Source: CAD feature listing. Evaluate the final solid. Frame: model axes, mm. Face numbers are marked on the shaded views. Give positions to 0.01 mm unless a question says otherwise; leave off trailing zeros. Write each loop counter-clockwise with the first axis right and the second up, starting at its lowest first coordinate (ties: lowest second). Pieces come first, ordered by that corner, then holes. Notation, with made-up numbers: (-29.5, 76.25) -> (-6.5, 76.25) arc R31 ccw to (-6.5, 110.25) -> close; hole circle Ø6 at (45.25, 3). An arc over 180 degrees is marked (long way). Write item = value, one per line.
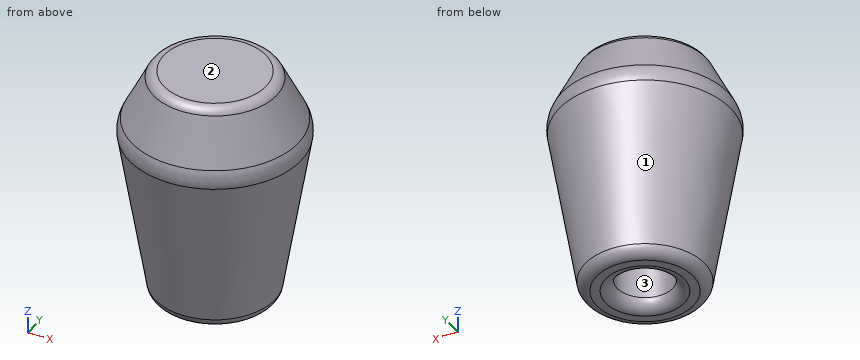
from build123d import *

# Parameters (mm, degrees)
F2_R     = 3.025775
F3_DEPTH = 11.43
F4_R     = 1.27
F5_R     = 3.175


with BuildPart() as f1:
    # F0 (on Front) → F1 (revolve)
    with BuildSketch(Plane.XZ):
        Polygon((0, 25.4), (0, 0), (6.35, 0), (9.525, 19.05), (6.35, 25.4), align=None)
    revolve(axis=Axis((0, 0, 12.7), (0, 0, 1)))

    # F2 (on face) → F3 (cut)
    with BuildSketch(Plane(origin=(0, 0, 0), x_dir=(1, 0, 0), z_dir=(0, 0, -1))):
        Circle(F2_R)
    extrude(amount=-F3_DEPTH, mode=Mode.SUBTRACT)

    # F4
    f4_edges = [f1.edges().sort_by_distance(p)[0] for p in [
        (-3.025775, 0, 0),
        (-6.35, 0, 25.4),
        (-6.35, 0, 0),
    ]]
    fillet(f4_edges, radius=F4_R)

    # F5
    f5_edges = [f1.edges().sort_by_distance(p)[0] for p in [
        (-9.525, 0, 19.05),
    ]]
    fillet(f5_edges, radius=F5_R)


solid = f1.part
(1) Section query B-B (z = 23.5). Return loops of the section in (x, y).
Values follow:
outline = circle Ø14.6 at (0, 0)
(2) Pull-direction query (X, two-part tool) for the marked faces 1, 2 and 3; classes: pulls with the +X half, pulls with the -X half, needs draft (parallel to the pull), parting line crosses it, or undercut.
Values follow:
face_1 = parting line crosses it
face_2 = needs draft
face_3 = undercut
(3) Material intervals for line 1 (X direction, y = 0, z = 5.5); line 2 (Z direction, x = -2.5, y = 1.5); line 3 (X direction, y = 0, z = 3.5), sorted ascending.
Values follow:
line_1 = -7.27 to -3.03, 3.03 to 7.27
line_2 = 11.43 to 25.4
line_3 = -6.93 to -3.03, 3.03 to 6.93
(4) Section query C-C (z = 3.75). Return loops of the section in (x, y) (3 decimals).
Values follow:
outline = circle Ø13.95 at (0, 0); hole circle Ø6.052 at (0, 0)
(5) First-contact query: pin 1 (1 mm diameter, centred on x = 3, z = 13, fed in from -Y); pin 2 (3 mm diameter, centred on x = -7, z = 17.5, fed in from +Y); pin 3 (5.5 mm diameter, centred on x = 0, y = 0, fed in from -Z). Flat tips, straight axial feed; report the tip coordinate or a pass-through.
Values follow:
pin_1 = -8.16
pin_2 = 7.5
pin_3 = 11.43
(6) Section query A-A (z = 10.5). Return loops of the section in (x, y).
Values follow:
outline = circle Ø16.2 at (0, 0); hole circle Ø6.05 at (0, 0)
